Geometry check sheet. Reference: drawing and pictorial views, mm from the part's lowest x, y, z. Give positions to 0.01 mm unless a question says otherwise; leave off trailing zeros. Write each loop counter-clockwise with the first axis right and the second up, starting at its lowest first coordinate (ties: lowest second). Pieces come first, ordered by that corner, then holes. Notation, with made-up numbers: M 12,12 L 23,12 A26 cw 23,50 Z; hole C 88,-6.5 d11. An arc over 180 degrees is marked long. Answer as a JSON object with one key per item and string values.
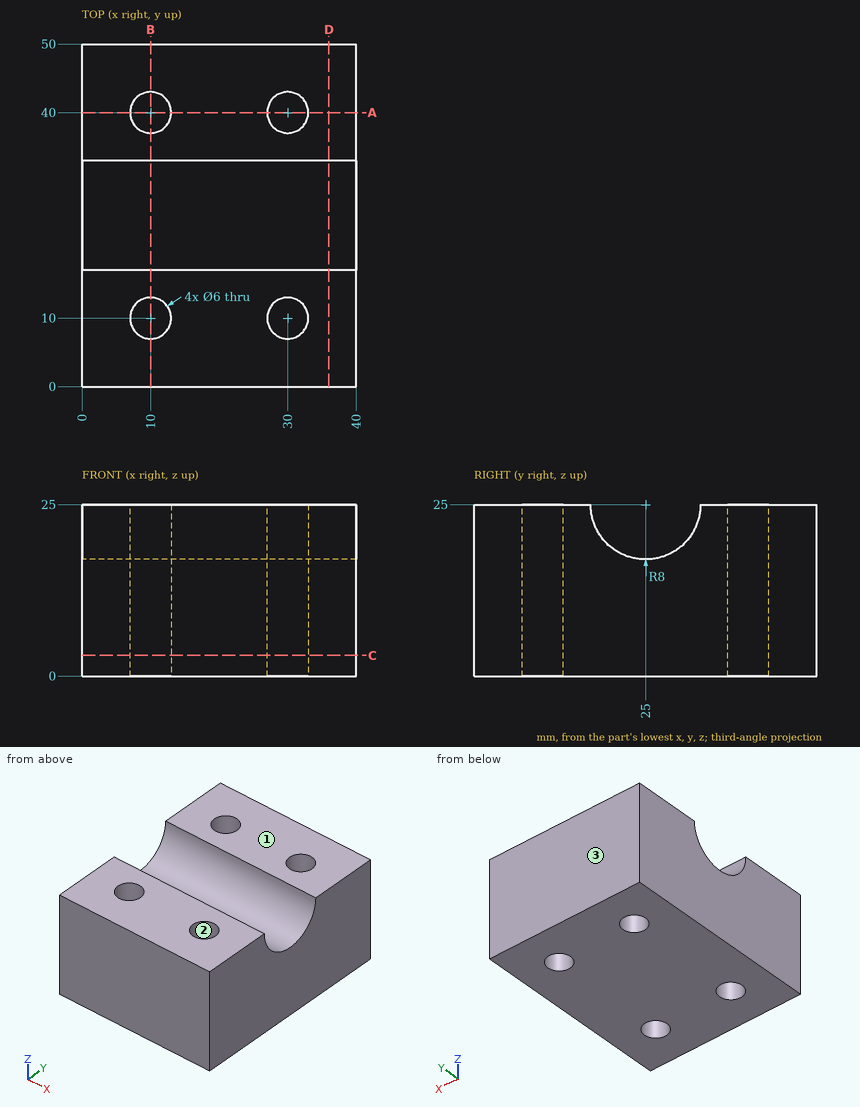
1) Section check B-B on x = 10. Record the boundary of the cut face in (y, z).
Completed:
{"outline": "M 0,0 L 7,0 L 7,25 L 0,25 Z; M 13,0 L 37,0 L 37,25 L 33,25 A8 cw 17,25 L 13,25 Z; M 43,0 L 50,0 L 50,25 L 43,25 Z"}
2) Section check A-A on y = 40. Record the boundary of the cut face in (x, z).
Completed:
{"outline": "M 0,0 L 7,0 L 7,25 L 0,25 Z; M 13,0 L 27,0 L 27,25 L 13,25 Z; M 33,0 L 40,0 L 40,25 L 33,25 Z"}
3) Section check D-D on x = 36. Record the boundary of the cut face in (y, z).
Completed:
{"outline": "M 0,0 L 50,0 L 50,25 L 33,25 A8 cw 17,25 L 0,25 Z"}
4) Section check C-C on z = 3. Record the boundary of the cut face in (x, y).
Completed:
{"outline": "M 0,0 L 40,0 L 40,50 L 0,50 Z; hole C 10,10 d6; hole C 10,40 d6; hole C 30,10 d6; hole C 30,40 d6"}
5) Release check for a two-part mould opening along Y. For the marked faces 1, 2 and 3 record: pulls with the +Y half, pulls with the -Y half, needs draft (parallel to the pull), parting line crosses it, or undercut.
Completed:
{"face 1": "needs draft", "face 2": "undercut", "face 3": "pulls with the +Y half"}
6) Thickness scan on L1, parallel to Y at x = 10, z = 14; L2, parallel to Y at x = 30, z = 18.5; L3, parallel to X at y = 37.5, z = 14.25. Record the ranges inside material, lowest first.
Completed:
{"L1": "y = 0 to 7, 13 to 37, 43 to 50", "L2": "y = 0 to 7, 13 to 20.34, 29.66 to 37, 43 to 50", "L3": "x = 0 to 8.34, 11.66 to 28.34, 31.66 to 40"}
7) Go/stop test with flat-tipped pins: pin 1 (12 mm diameter, centred on x = 13.5, y = 32, fed in from +Z); pin 2 (6 mm diameter, centred on x = 31.5, y = 22.5, fed in from +Z). Record where each tip stops, or that it passes through.
Completed:
{"pin 1": "stops at z = 25", "pin 2": "stops at z = 19.19"}
